Autodesk Inventor part; units mm, degrees
ref_plane "YZ Plane" through (0, 0, 0) normal (1, 0, 0) x (0, 1, 0)
ref_plane "XZ Plane" through (0, 0, 0) normal (0, 1, 0) x (-1, 0, 0)
ref_plane "XY Plane" through (0, 0, 0) normal (0, 0, 1) x (1, 0, 0)
sketch "Sketch1" plane through (0, 0, 0) normal (0, 1, 0) x (-1, 0, 0)
  circle A0 centre (0, 0) radius 6.35
  dimension "d0" = 12.7
extrude "Extrusion1" add sketch "Sketch1" along normal blind 25.4
hole "Hole1" at (0, 25.4, 0) direction (0, -1, 0) diameter 3.302 depth 9.525 tip angle 118
hole "Hole2" at (0, 0, 0) direction (0, 1, 0) diameter 3.302 depth 9.525 tip angle 118
properties part number "alumina_standoff_LSP_ASO00110"
Could you check a few things on this model? Use its own coordinates, in mm. A direction names the side the tool comes from. Coordinates: 2 decimals unless noted, no trailing zeros. Order: outer loops, then holes, each group sorted by start corner. A loop starts at its lowest first (then second) coordinate and runs counter-clockwise, first axis right, second up. Notation, with made-up numbers: (-2.5, -29.75) - (3.5, -29.75) arc R26 cw to (3.5, 8.25) - close; hole circle Ø5 at (0.25, 44.25). An arc over 180 degrees is marked (long way). Answer in a Markdown table with one row per item. Add a question column.
(1) On a 3-axis mill with a long thin cutter (end or side, diameter ignored), from which of +Z, -Z, +X, -X, +Y, -Y can I reach the whole of each face in a straight line? I mean faces 1 (the face through (0.632, 20.571, 1.525)), 2 (the face through (0.632, 4.829, -1.525)), 3 (the face through (-1.3, 0, -1.3)). Say none if no direction works.
(2) Will these pins go through, and if not, where does the flat tip stop? pin 1 (2.5 mm diameter, centred on x = 0, z = 0, fed in from -Y); pin 2 (1 mm diameter, centred on x = 3.5, y = 8.5, fed in from -Z); pin 3 (1.5 mm diameter, centred on y = 11, z = 2, fed in from -X).
(3) If we section it at D-D, the plane z = 5.5: Please give me the cut outline in (x, y), then the cut area to 3 significant figures.
(4) If we mould it in two halves opening along X, with no side actions, what happens to faces 4 (the face through (0.013, 15.055, -0.286)), 5 (the face through (-1.3, 25.4, -1.3)), 6 (the face through (1.38, 12.52, 6.2)), 7 (the face through (0.013, 10.345, 0.286))? For each: released by +X, released by -X, zero draft, split by the parting line, or undercut.
(5) If we section it at A-A, the plane y = 4.75: Please give me the cut outline in (x, z).
(6) If we section it at C-C, the plane y = 12.5: Please give me the cut outline in (x, z).
(7) If we section it at B-B, the plane z = 2.25: Please give me the cut outline in (x, y), then the cut area to 3 significant figures.
(8) I need wall thicknesses on L1, parallel to Z at x = 0, y = 18.75; L2, parallel to X at y = 1.5, z = 1.5; L3, parallel to Z at x = -1, y = 21.75. Which ranges of each line are inside material? Lowest first, please.
Results are:
| question | item | result |
|---|---|---|
| 1 | face 1 | +Y |
| 1 | face 2 | -Y |
| 1 | face 3 | +Z, -Z, +X, -X, -Y |
| 2 | pin 1 | stops at y = 9.77 |
| 2 | pin 2 | stops at z = -5.6 |
| 2 | pin 3 | stops at x = -6.23 |
| 3 | outline | (-3.17, 0) - (3.17, 0) - (3.17, 25.4) - (-3.17, 25.4) - close |
| 3 | area | 161 mm2 |
| 4 | face 4 | undercut |
| 4 | face 5 | zero draft |
| 4 | face 6 | split by the parting line |
| 4 | face 7 | undercut |
| 5 | outline | circle Ø12.7 at (0, 0); hole circle Ø3.3 at (0, 0) |
| 6 | outline | circle Ø12.7 at (0, 0) |
| 7 | outline | (-5.94, 0) - (5.94, 0) - (5.94, 25.4) - (-5.94, 25.4) - close |
| 7 | area | 302 mm2 |
| 8 | L1 | z = -6.35 to -1.65, 1.65 to 6.35 |
| 8 | L2 | x = -6.17 to -0.69, 0.69 to 6.17 |
| 8 | L3 | z = -6.27 to -1.31, 1.31 to 6.27 |
